Verification items for the finished model (mm, model axes). A direction names the side the tool comes from. Give positions to 0.01 mm unless a question says otherwise; leave off trailing zeros. Order: outer loops, then holes, each group sorted by start corner. A loop starts at its lowest first (then second) coordinate and runs counter-clockwise, first axis right, second up. Notation, with made-up numbers: (-22.5, 48) - (0.5, 48) arc R24 cw to (0.5, 74) - close; hole circle Ø8 at (74.25, -7.75). An arc over 180 degrees is marked (long way). Answer as a JSON object with one key per item and string values. Group by question number.
(1) Section check C-C (x = -4). Record the boundary of the cut face in (y, z), then the cut area to 3 significant figures.
(2) Mould release check, pull along X, two halves, no side actions. Record for faces 1 (the face through (-49.9, -55.3, 9.5)), 2 (the face through (-58.285, 58.373, 6.409)), 3 (the face through (53.37, 54.14, 11.73)), 4 (the face through (-1, -60, 6)): +X half, -X half, draft (parallel to the pull), parting line (faces both ways), or undercut.
(3) Thickness scan on line 1 (X direction, y = -52.03, z = 11.2); line 2 (Y direction, x = -52.03, z = 5.5); line 3 (Y direction, x = 52.5, z = 8). Record the ranges inside material, lowest first.
(4) Access from +Z, -Z, +X, -X, +Y, -Y to the whole of each face (thin tool, end or side, straight path). Record for faces 5 (the face through (-50.69, 54.14, 11.73)), 6 (the face through (0, 0, 1.5)), 7 (the face through (-47.411, -53.945, 4.684)).
(5) Depth check by flat-ended pin: pin 1 Ø3 at (x, y) = (52.03, -52.03) entering from +Z; pin 2 Ø5 at (x, y) = (51, -52.5) entering from -Z; pin 3 Ø6.5 at (x, y) = (-52.03, -52.03) entering from -Z; pin 4 Ø3 at (x, y) = (-52.5, -50.5) entering from -Z. Enter the tip coordinate at first touch or a pass-through.
(6) Section check A-A (x = 52.03). Record the boundary of the cut face in (y, z), then the cut area to 3 significant figures.
(7) Section check D-D (y = 0). Record the boundary of the cut face in (x, z), then the cut area to 3 significant figures.
```python
from build123d import *

# Parameters (mm, degrees)
F0_R     = 4.9999993943
F0_R_2   = 4.9999985195
F0_R_3   = 5
F0_R_4   = 21
F1_DEPTH = 13
F2_DEPTH = 1.5
F3_R     = 4.9999985195
F3_R_2   = 4.9999993943
F3_R_3   = 5
F4_DEPTH = 3.5
F0_R_5   = 2.5
F5_DEPTH = 27.6
F6_SIZE  = 1


with BuildPart() as f1:
    # F0 (on Top) → F1 (new body)
    with BuildSketch(Plane.XY):
        with BuildLine():
            Line((55, 60), (-54.2957481862, 60))
            ThreePointArc((-54.2957481862, 60), (-58.3292633253, 58.3292633253), (-60, 54.2957481862))
            Line((-60, 54.2957481862), (-60, -54.2957481862))
            ThreePointArc((-60, -54.2957481862), (-58.3292633253, -58.3292633253), (-54.2957481862, -60))
            Line((-54.2957481862, -60), (54.2957481862, -60))
            ThreePointArc((54.2957481862, -60), (58.3292633253, -58.3292633253), (60, -54.2957481862))
            Line((60, -54.2957481862), (60, 55))
            ThreePointArc((60, 55), (58.5355339059, 58.5355339059), (55, 60))
        make_face()
        with Locations((-52.03, -52.03)):
            Circle(F0_R, mode=Mode.SUBTRACT)
        with Locations((52.03, -52.03)):
            Circle(F0_R_2, mode=Mode.SUBTRACT)
        with Locations((-52.03, 52.03)):
            Circle(F0_R_3, mode=Mode.SUBTRACT)
        Circle(F0_R_4, mode=Mode.SUBTRACT)
        with Locations((52.03, 52.03)):
            Circle(F0_R_3, mode=Mode.SUBTRACT)
    extrude(amount=F1_DEPTH)

    # F0 (on Top) → F2 (join)
    with BuildSketch(Plane.XY):
        Circle(F0_R_4)
    extrude(amount=F2_DEPTH)

    # F3 (on face) → F4 (join)
    with BuildSketch(Plane.XY.offset(13)):
        with Locations((52.03, -52.03)):
            Circle(F3_R)
        with Locations((-52.03, -52.03)):
            Circle(F3_R_2)
        with Locations((-52.03, 52.03)):
            Circle(F3_R_3)
        with Locations((52.03, 52.03)):
            Circle(F3_R_3)
    extrude(amount=-F4_DEPTH)

    # F0 (on Top) → F5 (cut)
    with BuildSketch(Plane.XY):
        with Locations((-52.03, -52.03)):
            Circle(F0_R_5)
        with Locations((52.03, -52.03)):
            Circle(F0_R_5)
        with Locations((52.03, 52.03)):
            Circle(F0_R_5)
        with Locations((-52.03, 52.03)):
            Circle(F0_R_5)
    extrude(amount=F5_DEPTH, mode=Mode.SUBTRACT)

    # F6
    f6_edges = [f1.edges().sort_by_distance(p)[0] for p in [
        (49.53, 52.03, 9.5),
        (-54.53, 52.03, 9.5),
        (49.53, -52.03, 9.5),
        (-54.53, -52.03, 9.5),
    ]]
    chamfer(f6_edges, length=F6_SIZE)


solid = f1.part
```
Solutions:
{
 "1": {"outline": "(-60, 0) - (60, 0) - (60, 13) - (20.62, 13) - (20.62, 1.5) - (-20.62, 1.5) - (-20.62, 13) - (-60, 13) - close", "area": "1,090 mm2"},
 "2": {"face 1": "undercut", "face 2": "-X half", "face 3": "undercut", "face 4": "draft"},
 "3": {"line 1": "x = -60 to -54.53, -49.53 to 49.53, 54.53 to 60", "line 2": "y = -60 to -57.03, -47.03 to 47.03, 57.03 to 60", "line 3": "y = -60 to -57.01, -47.05 to 47.05, 57.01 to 60"},
 "4": {"face 5": "+Z, -Z", "face 6": "+Z", "face 7": "-Z"},
 "5": {"pin 1": "passes through", "pin 2": "stops at z = 9.5", "pin 3": "stops at z = 9.75", "pin 4": "stops at z = 9.9"},
 "6": {"outline": "(-60, 0) - (-57.03, 0) - (-57.03, 9.5) - (-55.53, 9.5) - (-54.53, 10.5) - (-54.53, 13) - (-60, 13) - close; (-49.53, 10.5) - (-48.53, 9.5) - (-47.03, 9.5) - (-47.03, 0) - (47.03, 0) - (47.03, 9.5) - (48.53, 9.5) - (49.53, 10.5) - (49.53, 13) - (-49.53, 13) - close; (54.53, 10.5) - (55.53, 9.5) - (57.03, 9.5) - (57.03, 0) - (60, 0) - (60, 13) - (54.53, 13) - close", "area": "1,330 mm2"},
 "7": {"outline": "(-60, 0) - (60, 0) - (60, 13) - (21, 13) - (21, 1.5) - (-21, 1.5) - (-21, 13) - (-60, 13) - close", "area": "1,080 mm2"}
}
